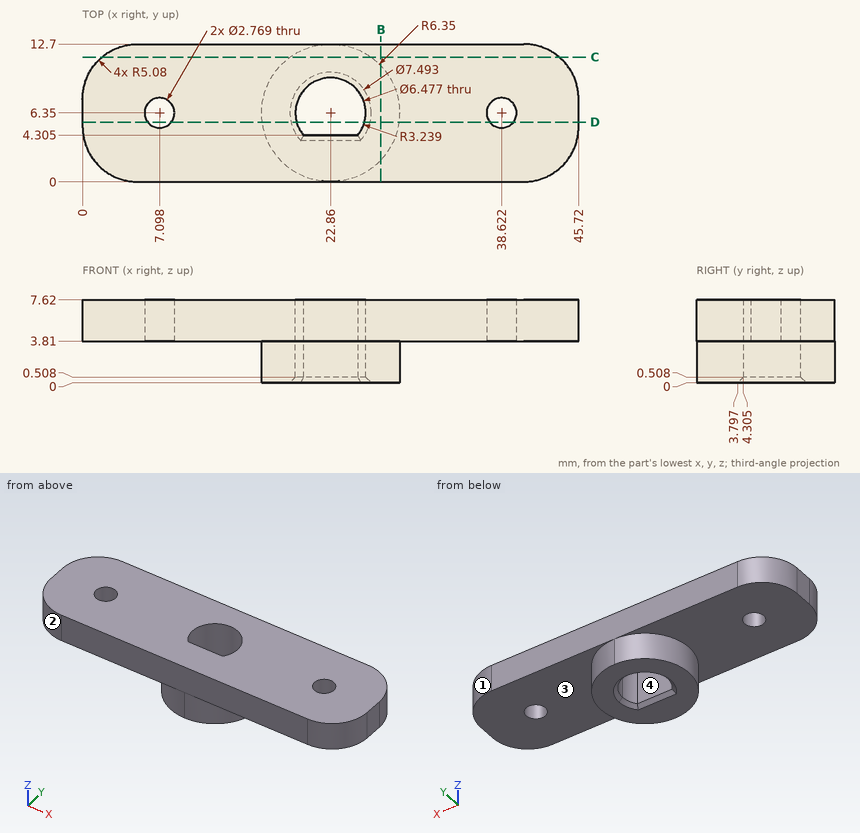
Input: dimensioned drawing with shaded views. Units: mm. Origin: part minimum x, y, z. Round coordinates to 2 decimals unless told otherwise and drop trailing zeros. Loops run counter-clockwise (first coordinate to the right, second up) from the corner with the lowest first, then second, coordinate; pieces in that order, holes last. Notation, with made-up numbers: (49, 83) -> (108, 83) arc R34 cw to (108, 120) -> close; hole circle Ø2 at (42, 31). An arc over 180 degrees is marked (long way). Answer as a JSON object with one key per item and string values. Group by question number.
1) Draft query along Y for the marked faces 1, 2, 3 and 4. Return one class per face: +Y half, -Y half, draft (parallel to the pull), parting line (faces both ways), or undercut.
2) Section query D-D on y = 5.5. State how many separate pieces and enclosed holes the cut face has.
3) Section query C-C on y = 11.5. Output: boundary loops of the cut face in (x, z) (1 decimal).
4) Ray query, L1, parallel to Y at x = 22.86, z = 4 (1 decimal); L2, parallel to X at y = 5.5, z = 4.5 (1 decimal); L3, parallel to Z at x = 16.5, y = 5.25. Return the intervals inside material, ascending.
5) Pin query (flat end, axial travel): pin 1 (2 mm diameter, centred on x = 38.62, y = 6.35, fed in from +Z); pin 2 (1 mm diameter, centred on y = 11, z = 2.5, fed in from +X) (1 decimal); pin 3 (1 mm diameter, centred on x = 16, y = 11.5, fed in from -Z); pin 4 (1 mm diameter, centred on y = 4.5, z = 5.5, fed in from -X). Return the tip coordinate at first contact, or that it passes through.
6) Section query B-B on x = 27.5. Output: boundary loops of the cut face in (y, z) (1 decimal).
Reply:
{
 "1": {"face 1": "+Y half", "face 2": "-Y half", "face 3": "draft", "face 4": "undercut"},
 "2": {"separate pieces": "4", "enclosed holes": "0"},
 "3": {"outline": "(1.8, 3.8) -> (19.1, 3.8) -> (19.1, 0) -> (26.6, 0) -> (26.6, 3.8) -> (43.9, 3.8) -> (43.9, 7.6) -> (1.8, 7.6) -> close"},
 "4": {"L1": "y = 0 to 4.3, 9.6 to 12.7", "L2": "x = 0 to 6, 8.2 to 19.7, 26 to 37.5, 39.7 to 45.7", "L3": "z = 3.81 to 7.62"},
 "5": {"pin 1": "passes through", "pin 2": "stops at x = 27.7", "pin 3": "stops at z = 3.81", "pin 4": "stops at x = 0"},
 "6": {"outline": "(0, 3.8) -> (2, 3.8) -> (2, 0) -> (10.7, 0) -> (10.7, 3.8) -> (12.7, 3.8) -> (12.7, 7.6) -> (0, 7.6) -> close"}
}
